Drawing for the job (mm, zero at the part's lowest x, y, z). Give positions to 0.01 mm unless a question says otherwise; leave off trailing zeros. Order: outer loops, then holes, each group sorted by start corner. A loop starts at its lowest first (then second) coordinate and runs counter-clockwise, first axis right, second up. Notation, with made-up numbers: (8.5, 15.5) - (35.5, 15.5) arc R25 cw to (35.5, 32.5) - close; hole circle Ø1 at (-15.5, 73.5). An arc over 180 degrees is marked (long way). One line per item, written item: value.
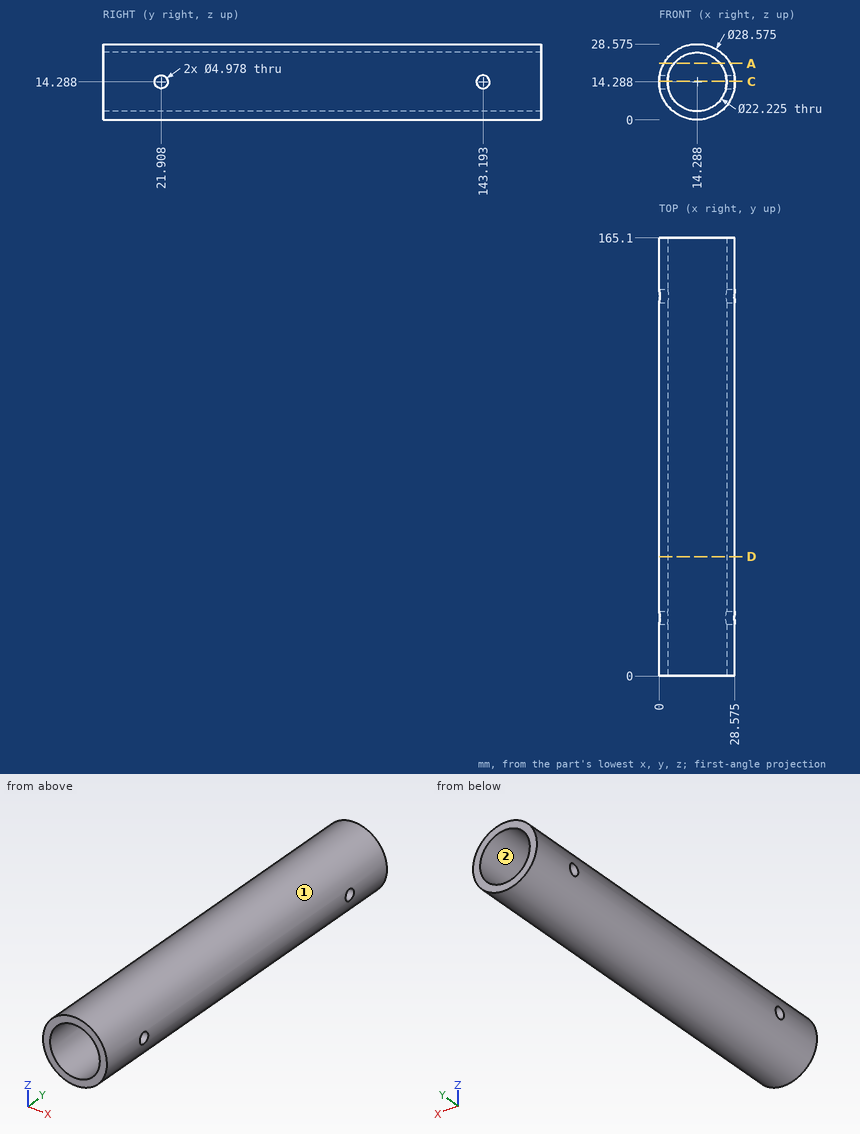
(1) Slice it at D-D, the plane y = 45. Give the cut face in (x, z) (1 decimal).
Completed:
outline: circle Ø28.6 at (14.3, 14.3); hole circle Ø22.2 at (14.3, 14.3)
(2) Slice it at C-C, the plane z = 14.5. Give the cut face in (x, y).
Completed:
outline: (0, 0) - (3.18, 0) - (3.18, 19.43) - (0, 19.43) - close; (0, 24.39) - (3.18, 24.39) - (3.18, 140.71) - (0, 140.71) - close; (0, 145.67) - (3.18, 145.67) - (3.18, 165.1) - (0, 165.1) - close; (25.4, 0) - (28.57, 0) - (28.57, 19.43) - (25.4, 19.43) - close; (25.4, 24.39) - (28.57, 24.39) - (28.57, 140.71) - (25.4, 140.71) - close; (25.4, 145.67) - (28.57, 145.67) - (28.57, 165.1) - (25.4, 165.1) - close
(3) Slice it at A-A, the plane z = 21.25. Give the cut face in (x, y).
Completed:
outline: (1.81, 0) - (5.63, 0) - (5.63, 165.1) - (1.81, 165.1) - close; (22.95, 0) - (26.76, 0) - (26.76, 165.1) - (22.95, 165.1) - close
(4) Pull direction X, two halves, no side cores. Call the marked faces 1 and 2: +X half, -X half, draft (parallel to the pull), parting line (faces both ways), or undercut.
Completed:
face 1: parting line
face 2: undercut
(5) Pin check, flat tips, straight feed: P1, Ø13.5, axis at x = 14.29, z = 14.29, coming from the +Y side; P2, Ø1.5, axis at x = 3, y = 134, coming from the -Z side; P3, Ø1, axis at x = 19.5, y = 106, coming from the +Z side (1 decimal); P4, Ø4, axis at x = 11, y = 119.5, coming from the -Z side. Stop position of each tip, or through.
Completed:
P1: through
P2: z = 4.64
P3: z = 27.8
P4: z = 0.06
(6) Drill centre lines: line 1 (Z direction, x = 14.75, y = 150.5) (1 decimal); line 2 (X direction, y = 18, z = 14.5); line 3 (X direction, y = 10, z = 7.25) (1 decimal). Where is each one in solid material? Low to high.
Completed:
line 1: 0 to 3.2, 25.4 to 28.6
line 2: 0 to 3.18, 25.4 to 28.57
line 3: 1.9 to 5.7, 22.9 to 26.7
